Read the model definition and answer for the solid it produces. Units are mm, in the model's axes. A direction names the side the tool comes from. Coordinates: 2 decimals unless noted, no trailing zeros. Write each loop counter-clockwise with the first axis right and the second up, starting at its lowest first coordinate (ties: lowest second). Pieces come first, ordered by that corner, then holes. Notation, with made-up numbers: (47.5, 74.5) -> (66.5, 74.5) arc R23 cw to (66.5, 84.5) -> close; hole circle Ø4 at (-32.5, 17). An arc over 180 degrees is marked (long way). Answer as a JSON object with one key per item and string values. Group by question number.
(1) Flat-ended cylindrical pins translate along their axes: P1, Ø5, axis at y = 68.5, z = 51, coming from the +X side; P2, Ø19, axis at x = 27.5, z = 38, coming from the +Y side; P3, Ø6.5, axis at x = 23.55, z = 75, coming from the +Y side. Find the tip coordinate at first contact, or state that the pin passes through.
(2) For a pull along Y with two mould halves and no side action, classify faces 1 (the face through (7.395, 82.859, 44.673)), 2 (the face through (7.395, 63.483, 54.757)), 3 (the face through (7, 0, 49)), 4 (the face through (-9.04, 3.04, 12.56)) as +Y half, -Y half, draft (parallel to the pull), parting line (faces both ways), or undercut.
(3) Find section C-C (z = 93.5). Give the vertices of the cut face in (x, y).
(4) Find section A-A (z = 15). Give the vertices of the cut face in (x, y).
(5) Straight lines are drawn through the part: L1, parallel to X at y = 3, z = 75; L2, parallel to Z at x = 23.55, y = 4.5; L3, parallel to Y at x = 11, z = 91. For each, find the intervals that lie inside material, in ascending order.
(6) Which of the six approach directions +Z, -Z, +X, -X, +Y, -Y give full straight-line access (tool end or side, diameter ignored) to faces 5 (the face through (7, 63, 70)), 6 (the face through (7, 168, 95)), 7 (the face through (15, 2, 95)), 8 (the face through (0, 2, 95))?
(7) Find section B-B (x = -8.5). Give the vertices of the cut face in (y, z).
(8) Find section D-D (x = 9). Give the vertices of the cut face in (y, z).
from build123d import *

# Parameters (mm, degrees)
CYLINDER005_R          = 2.5
CYLINDER005_DEPTH      = 20
CYLINDER005_ROLL_ANGLE = 90
CYLINDER004_R          = 2.5
CYLINDER004_DEPTH      = 20
CYLINDER004_ROLL_ANGLE = 90
CYLINDER003_R          = 2.5
CYLINDER003_DEPTH      = 20
CYLINDER003_ROLL_ANGLE = 90
CYLINDER002_R          = 2.5
CYLINDER002_DEPTH      = 20
CYLINDER002_ROLL_ANGLE = 90
CYLINDER001_R          = 2.5
CYLINDER001_DEPTH      = 20
CYLINDER001_ROLL_ANGLE = 90
CYLINDER_R             = 2.5
CYLINDER_DEPTH         = 20
CYLINDER_ROLL_ANGLE    = 90
BOX002_W               = 15
BOX002_H               = 163
BOX002_DEPTH           = 100
BOX003_W               = 15
BOX003_H               = 125
BOX003_DEPTH           = 18
BOX003_ROLL_ANGLE      = 28
BOX001_W               = 15
BOX001_H               = 163
BOX001_DEPTH           = 100
BOX_W                  = 15
BOX_H                  = 173
BOX_DEPTH              = 100
CHAMFER001_SIZE        = 4
BOX004_W               = 50
BOX004_H               = 8
BOX004_DEPTH           = 90
CHAMFER_SIZE           = 4
CHAMFER002_SIZE        = 4
CHAMFER003_SIZE        = 2


with BuildPart() as cylinder005:
    # Cylinder005 → Cylinder005 (new body)
    with BuildSketch(Plane.XY):
        Circle(CYLINDER005_R)
    extrude(amount=CYLINDER005_DEPTH)


with BuildPart() as cylinder005_1:
    # Cylinder005 roll: moved
    add(cylinder005.part.rotate(Axis((0, 0, 0), (1, 0, 0)), CYLINDER005_ROLL_ANGLE))


with BuildPart() as cylinder005_2:
    # Cylinder005 placement: moved
    add(cylinder005_1.part.moved(Location((-8.5, 14, 75))))


with BuildPart() as cylinder004:
    # Cylinder004 → Cylinder004 (new body)
    with BuildSketch(Plane.XY):
        Circle(CYLINDER004_R)
    extrude(amount=CYLINDER004_DEPTH)


with BuildPart() as cylinder004_1:
    # Cylinder004 roll: moved
    add(cylinder004.part.rotate(Axis((0, 0, 0), (1, 0, 0)), CYLINDER004_ROLL_ANGLE))


with BuildPart() as cylinder004_2:
    # Cylinder004 placement: moved
    add(cylinder004_1.part.moved(Location((23.55, 14, 75))))


with BuildPart() as cylinder003:
    # Cylinder003 → Cylinder003 (new body)
    with BuildSketch(Plane.XY):
        Circle(CYLINDER003_R)
    extrude(amount=CYLINDER003_DEPTH)


with BuildPart() as cylinder003_1:
    # Cylinder003 roll: moved
    add(cylinder003.part.rotate(Axis((0, 0, 0), (1, 0, 0)), CYLINDER003_ROLL_ANGLE))


with BuildPart() as cylinder003_2:
    # Cylinder003 placement: moved
    add(cylinder003_1.part.moved(Location((-8.5, 14, 45))))


with BuildPart() as cylinder002:
    # Cylinder002 → Cylinder002 (new body)
    with BuildSketch(Plane.XY):
        Circle(CYLINDER002_R)
    extrude(amount=CYLINDER002_DEPTH)


with BuildPart() as cylinder002_1:
    # Cylinder002 roll: moved
    add(cylinder002.part.rotate(Axis((0, 0, 0), (1, 0, 0)), CYLINDER002_ROLL_ANGLE))


with BuildPart() as cylinder002_2:
    # Cylinder002 placement: moved
    add(cylinder002_1.part.moved(Location((23.55, 14, 45))))


with BuildPart() as cylinder001:
    # Cylinder001 → Cylinder001 (new body)
    with BuildSketch(Plane.XY):
        Circle(CYLINDER001_R)
    extrude(amount=CYLINDER001_DEPTH)


with BuildPart() as cylinder001_1:
    # Cylinder001 roll: moved
    add(cylinder001.part.rotate(Axis((0, 0, 0), (1, 0, 0)), CYLINDER001_ROLL_ANGLE))


with BuildPart() as cylinder001_2:
    # Cylinder001 placement: moved
    add(cylinder001_1.part.moved(Location((-8.5, 14, 15))))


with BuildPart() as cylinder:
    # Cylinder → Cylinder (new body)
    with BuildSketch(Plane.XY):
        Circle(CYLINDER_R)
    extrude(amount=CYLINDER_DEPTH)


with BuildPart() as cylinder_1:
    # Cylinder roll: moved
    add(cylinder.part.rotate(Axis((0, 0, 0), (1, 0, 0)), CYLINDER_ROLL_ANGLE))


with BuildPart() as cylinder_2:
    # Cylinder placement: moved
    add(cylinder_1.part.moved(Location((23.55, 14, 15))))


with BuildPart() as cube002:
    # Box002 → Box002 (new body)
    with BuildSketch(Plane(origin=(0, 5, 90), x_dir=(1, 0, 0), z_dir=(0, 0, 1))):
        with Locations((7.5, 81.5)):
            Rectangle(BOX002_W, BOX002_H)
    extrude(amount=BOX002_DEPTH)


with BuildPart() as cube003:
    # Box003 → Box003 (new body)
    with BuildSketch(Plane.XY):
        with Locations((7.5, 62.5)):
            Rectangle(BOX003_W, BOX003_H)
    extrude(amount=BOX003_DEPTH)


with BuildPart() as cube003_1:
    # Box003 roll: moved
    add(cube003.part.rotate(Axis((0, 0, 0), (1, 0, 0)), BOX003_ROLL_ANGLE))


with BuildPart() as cube003_2:
    # Box003 placement: moved
    add(cube003_1.part.moved(Location((0, 20, 11.25))))


with BuildPart() as cube001:
    # Box001 → Box001 (new body)
    with BuildSketch(Plane(origin=(0, 34, -30), x_dir=(1, 0, 0), z_dir=(0, 0, 1))):
        with Locations((7.5, 81.5)):
            Rectangle(BOX001_W, BOX001_H)
    extrude(amount=BOX001_DEPTH)


with BuildPart() as chamfer001:
    # Box → Box (new body)
    with BuildSketch(Plane.XY):
        with Locations((7.5, 86.5)):
            Rectangle(BOX_W, BOX_H)
    extrude(amount=BOX_DEPTH)

    # Cut: cut Cube001
    add(cube001.part, mode=Mode.SUBTRACT)

    # Fusion: union Cube003
    add(cube003_2.part)

    # Chamfer001
    chamfer001_edges = [chamfer001.edges().sort_by_distance(p)[0] for p in [
        (7.5, 34, 0),
    ]]
    chamfer(chamfer001_edges, length=CHAMFER001_SIZE)


with BuildPart() as final:
    # Box004 → Box004 (new body)
    with BuildSketch(Plane(origin=(-17.5, 0, 0), x_dir=(1, 0, 0), z_dir=(0, 0, 1))):
        with Locations((25, 4)):
            Rectangle(BOX004_W, BOX004_H)
    extrude(amount=BOX004_DEPTH)

    # Chamfer
    chamfer_edges = [final.edges().sort_by_distance(p)[0] for p in [
        (-17.5, 4, 90),
        (-17.5, 4, 0),
        (32.5, 4, 90),
        (32.5, 4, 0),
    ]]
    chamfer(chamfer_edges, length=CHAMFER_SIZE)

    # Fusion001: union Chamfer001
    add(chamfer001.part)

    # Cut001: cut Cube002
    add(cube002.part, mode=Mode.SUBTRACT)

    # Chamfer002
    chamfer002_edges = [final.edges().sort_by_distance(p)[0] for p in [
        (7.5, 173, 70),
    ]]
    chamfer(chamfer002_edges, length=CHAMFER002_SIZE)

    # Cut002: cut Cylinder
    add(cylinder_2.part, mode=Mode.SUBTRACT)

    # Cut003: cut Cylinder001
    add(cylinder001_2.part, mode=Mode.SUBTRACT)

    # Cut004: cut Cylinder002
    add(cylinder002_2.part, mode=Mode.SUBTRACT)

    # Cut005: cut Cylinder003
    add(cylinder003_2.part, mode=Mode.SUBTRACT)

    # Cut006: cut Cylinder004
    add(cylinder004_2.part, mode=Mode.SUBTRACT)

    # Cut007: cut Cylinder005
    add(cylinder005_2.part, mode=Mode.SUBTRACT)

    # Chamfer003
    chamfer003_edges = [final.edges().sort_by_distance(p)[0] for p in [
        (-11, 8, 75),
        (-11, 8, 45),
        (-11, 8, 15),
        (21.05, 8, 75),
        (21.05, 8, 45),
        (21.05, 8, 15),
    ]]
    chamfer(chamfer003_edges, length=CHAMFER003_SIZE)


solid = final.part
Results below:
{
 "1": {"P1": "stops at x = 15", "P2": "stops at y = 8", "P3": "stops at y = 6.75"},
 "2": {"face 1": "+Y half", "face 2": "undercut", "face 3": "-Y half", "face 4": "draft"},
 "3": {"outline": "(0, 0) -> (15, 0) -> (15, 5) -> (0, 5) -> close; (0, 168) -> (15, 168) -> (15, 173) -> (0, 173) -> close"},
 "4": {"outline": "(-17.5, 0) -> (-11, 0) -> (-11, 6) -> (-13, 8) -> (-17.5, 8) -> close; (-6, 0) -> (21.05, 0) -> (21.05, 6) -> (19.05, 8) -> (15, 8) -> (15, 34) -> (0, 34) -> (0, 8) -> (-4, 8) -> (-6, 6) -> close; (26.05, 0) -> (32.5, 0) -> (32.5, 8) -> (28.05, 8) -> (26.05, 6) -> close"},
 "5": {"L1": "x = -17.5 to -11, -6 to 21.05, 26.05 to 32.5", "L2": "z = 0 to 12.5, 17.5 to 42.5, 47.5 to 72.5, 77.5 to 90", "L3": "y = 0 to 5, 168 to 173"},
 "6": {"face 5": "+X, -X", "face 6": "+Z, +X, -X", "face 7": "+Z, +X, +Y, -Y", "face 8": "+Z, -X, +Y, -Y"},
 "7": {"outline": "(0, 0) -> (8, 0) -> (8, 10.5) -> (6, 12.5) -> (0, 12.5) -> close; (0, 17.5) -> (6, 17.5) -> (8, 19.5) -> (8, 40.5) -> (6, 42.5) -> (0, 42.5) -> close; (0, 47.5) -> (6, 47.5) -> (8, 49.5) -> (8, 70.5) -> (6, 72.5) -> (0, 72.5) -> close; (0, 77.5) -> (6, 77.5) -> (8, 79.5) -> (8, 90) -> (0, 90) -> close"},
 "8": {"outline": "(0, 0) -> (30, 0) -> (34, 4) -> (34, 18.69) -> (130.37, 69.93) -> (130.33, 70) -> (169, 70) -> (173, 74) -> (173, 100) -> (168, 100) -> (168, 90) -> (5, 90) -> (5, 100) -> (0, 100) -> close; hole (34, 39.08) -> (92.15, 70) -> (34, 70) -> close"}
}
